from build123d import *

# Parameters (mm, degrees)
F0_R      = 50
F1_DEPTH  = 40
F2_R      = 45
F3_DEPTH  = 35
F4_W      = 10
F4_H      = 6
F5_DEPTH  = 50
F6_W      = 10
F6_H      = 6
F7_DEPTH  = 50
F8_W      = 10
F8_H      = 5.49967
F9_DEPTH  = 50
F10_W     = 10
F10_H     = 5.49967
F11_DEPTH = 50


with BuildPart() as f1:
    # F0 (on Top) → F1 (new body)
    with BuildSketch(Plane.XY):
        Circle(F0_R)
    extrude(amount=F1_DEPTH)

    # F2 (on face) → F3 (cut)
    with BuildSketch(Plane.XY.offset(40)):
        Circle(F2_R)
    extrude(amount=-F3_DEPTH, mode=Mode.SUBTRACT)

    # F4 (on Front) → F5 (cut)
    with BuildSketch(Plane.XZ):
        with Locations((0, 37)):
            Rectangle(F4_W, F4_H)
    extrude(amount=-F5_DEPTH, mode=Mode.SUBTRACT)

    # F6 (on Front) → F7 (cut)
    with BuildSketch(Plane.XZ):
        with Locations((0, 37)):
            Rectangle(F6_W, F6_H)
    extrude(amount=F7_DEPTH, mode=Mode.SUBTRACT)

    # F8 (on Right) → F9 (cut)
    with BuildSketch(Plane.YZ):
        with Locations((0, 37.250165)):
            Rectangle(F8_W, F8_H)
    extrude(amount=-F9_DEPTH, mode=Mode.SUBTRACT)

    # F10 (on Right) → F11 (cut)
    with BuildSketch(Plane.YZ):
        with Locations((0, 37.250165)):
            Rectangle(F10_W, F10_H)
    extrude(amount=F11_DEPTH, mode=Mode.SUBTRACT)


solid = f1.part
Design review of the part built by this model. Coordinates are the model's own, in mm. A direction names the side the tool comes from. Coordinates: 2 decimals unless noted, no trailing zeros. Loops run counter-clockwise (first coordinate to the right, second up) from the corner with the lowest first, then second, coordinate; pieces in that order, holes last. Notation, with made-up numbers: (65, 34) - (117, 34) arc R21 cw to (117, 53) - close; hole circle Ø9 at (20.5, 79). An arc over 180 degrees is marked (long way). Use CSV: the item, a comma, the result in double quotes. Start each with the question number.
1. Add section B-B on x = 0. Give the boundary of the cut face in (y, z), plus the area to 3 significant figures.
2. For faces 1 (the flat face through (47, 5, 37)), 2 (the flat face through (-1, 1, 5)), 3 (the flat face through (5, 47, 37)), list the 3-axis set-ups (+Z, -Z, +X, -X, +Y, -Y) from which the entire face can be reached by the end or side of a thin tool; tool diameter is ignored.
3. To check wall thickness, follow probe 1 along X at (y, z) = (0, 18.5); probe 2 along Z at (x, y) = (22, -26). State the ranges of each line that lie inside material, in increasing order.
4. Clearance check with flat-ended pins moving along their axes: pin 1 (1.5 mm diameter, centred on y = 8, z = 7.5, fed in from -X); pin 2 (5.5 mm diameter, centred on x = 46.5, z = 38.5, fed in from -Y); pin 3 (2.5 mm diameter, centred on x = -48.5, y = -2, fed in from +Z); pin 4 (1.5 mm diameter, centred on x = -33, y = -15.5, fed in from -Z). State where each tip first meets the part, or that it passes through.
5. Add section A-A on y = 0. Give the boundary of the cut face in (x, z).
6. Add section C-C on z = 10.5. Give the boundary of the cut face in (x, y).
Resolved:
1,outline,"(-50, 0) - (50, 0) - (50, 34) - (45, 34) - (45, 5) - (-45, 5) - (-45, 34) - (-50, 34) - close"
1,area,"790 mm2"
2,face 1,"+Z, +X, -X"
2,face 2,"+Z"
2,face 3,"+Z, +Y, -Y"
3,probe 1,"-50 to -45, 45 to 50"
3,probe 2,"0 to 5"
4,pin 1,"x = -49.47"
4,pin 2,"y = -24.21"
4,pin 3,"z = 34.5"
4,pin 4,"z = 0"
5,outline,"(-50, 0) - (50, 0) - (50, 34.5) - (45, 34.5) - (45, 5) - (-45, 5) - (-45, 34.5) - (-50, 34.5) - close"
6,outline,"circle Ø100 at (0, 0); hole circle Ø90 at (0, 0)"
